```python
from build123d import *

# Parameters (mm, degrees)
F0_W     = 330.2
F0_H     = 254
F1_DEPTH = 7.62
F2_R     = 38.1
F4_DEPTH = 7.621
F3_R     = 19.05
F5_DEPTH = 7.621


with BuildPart() as f1:
    # F0 (on Top) → F1 (new body)
    with BuildSketch(Plane.XY):
        with Locations((-0.02661, -0.518168)):
            Rectangle(F0_W, F0_H)
    extrude(amount=F1_DEPTH)

    # F2 (on face) → F4 (cut, through all)
    with BuildSketch(Plane.XY.offset(7.62)):
        Circle(F2_R)
    extrude(amount=-F4_DEPTH, mode=Mode.SUBTRACT)

    # F3 (on face) → F5 (cut, through all)
    with BuildSketch(Plane.XY.offset(7.62)):
        with Locations((-133.37661, 0)):
            Circle(F3_R)
    extrude(amount=-F5_DEPTH, mode=Mode.SUBTRACT)


solid = f1.part
```
Geometry check sheet. Reference: the model listing, model coordinates, mm. Round coordinates to 2 decimals unless told otherwise and drop trailing zeros. Loops run counter-clockwise (first coordinate to the right, second up) from the corner with the lowest first, then second, coordinate; pieces in that order, holes last. Notation, with made-up numbers: M -23.75,56.5 L -18.75,56.5 A25 ccw -18.75,87.5 Z; hole C 40.25,75 d11. An arc over 180 degrees is marked long. Return JSON: item names as keys, results as strings. Group by question number.
(1) Mould release check, pull along X, two halves, no side actions. Record for faces 1 (the face through (-39, 1, 0)), 2 (the face through (165.073, -2, 4)), 3 (the face through (-30.235, -23.183, 3.863)): pulls with the +X half, pulls with the -X half, needs draft (parallel to the pull), parting line crosses it, or undercut.
(2) Section check C-C, the plane z = 3.75. Enter the section's corners in (x, y).
(3) Section check A-A, the plane y = 0. Enter the section's corners in (x, z).
(4) Section check B-B, the plane x = 0. Enter the section's corners in (y, z).
(5) Section check D-D, the plane y = -31.5. Enter the section's corners in (x, z), and give its area (3 significant figures).
(6) Scan lines: line 1 along Y through (x, z) = (-124, 5); line 2 along Y through (x, z) = (-128, 0.5); line 3 along X through (y, z) = (-33.5, 7). Record each from-to range of solid material in increasing order. Write a range as [from, to].
Data:
{
 "1": {"face 1": "needs draft", "face 2": "pulls with the +X half", "face 3": "undercut"},
 "2": {"outline": "M -165.13,-127.52 L 165.07,-127.52 L 165.07,126.48 L -165.13,126.48 Z; hole C -133.38,0 d38.1; hole C 0,0 d76.2"},
 "3": {"outline": "M -165.13,0 L -152.43,0 L -152.43,7.62 L -165.13,7.62 Z; M -114.33,0 L -38.1,0 L -38.1,7.62 L -114.33,7.62 Z; M 38.1,0 L 165.07,0 L 165.07,7.62 L 38.1,7.62 Z"},
 "4": {"outline": "M -127.52,0 L -38.1,0 L -38.1,7.62 L -127.52,7.62 Z; M 38.1,0 L 126.48,0 L 126.48,7.62 L 38.1,7.62 Z"},
 "5": {"outline": "M -165.13,0 L -21.43,0 L -21.43,7.62 L -165.13,7.62 Z; M 21.43,0 L 165.07,0 L 165.07,7.62 L 21.43,7.62 Z", "area": "2,190 mm²"},
 "6": {"line 1": "[-127.52, -16.58], [16.58, 126.48]", "line 2": "[-127.52, -18.28], [18.28, 126.48]", "line 3": "[-165.13, -18.15], [18.15, 165.07]"}
}
